```python
from build123d import *

# Parameters (mm, degrees)
ESQUISSE1_R                 = 20.5
ESQUISSE1_R_2               = 18.5
BOSS_EXTRU_1_DEPTH          = 20
BOSS_EXTRU_2_START          = 10
ESQUISSE2_R                 = 20.5
BOSS_EXTRU_2_DEPTH          = 10
BOSS_EXTRU_4_DEPTH          = 5
BOSS_EXTRU_5_DEPTH          = 10
TROU_TARAUD_M41_D           = 3.3
TROU_TARAUD_M41_CSINK_D     = 4.05
TROU_TARAUD_M41_CSINK_ANGLE = 90


with BuildPart() as part:
    # Esquisse1 → Boss.-Extru.1 (new body)
    with BuildSketch(Plane.XY):
        Circle(ESQUISSE1_R)
        Circle(ESQUISSE1_R_2, mode=Mode.SUBTRACT)
    extrude(amount=BOSS_EXTRU_1_DEPTH)

    # Esquisse2 → Boss.-Extru.2 (add)
    with BuildSketch(Plane(origin=(0, 0, 0), x_dir=(-1, 0, 0), z_dir=(0, 0, -1)).offset(BOSS_EXTRU_2_START)):
        Circle(ESQUISSE2_R)
    extrude(amount=-BOSS_EXTRU_2_DEPTH)



with BuildPart() as body_2:
    # Esquisse5 → Boss.-Extru.4 (new body)
    with BuildSketch(Plane(origin=(0, 20.5, 0), x_dir=(1, 0, 0), z_dir=(0, 1, 0))):
        Polygon((0, 0), (40, 0), (40, 10), (10, 10), (-40, 10), (-40, 0), align=None)
    extrude(amount=BOSS_EXTRU_4_DEPTH)


with BuildPart() as part_1:
    add(part.part)

    add(body_2.part)  # Boss.-Extru.5 merges body 2
    # Esquisse7 → Boss.-Extru.5 (add)
    with BuildSketch(Plane.XY.offset(-10)):
        with BuildLine():
            ThreePointArc((20.5, 0), (14.495689014, 14.495689014), (0, 20.5))
            Line((0, 20.5), (20.5, 20.5))
            Line((20.5, 20.5), (20.5, 0))
        make_face()
        with BuildLine():
            Line((-20.5, 20.5), (-20.5, 0))
            ThreePointArc((-20.5, 0), (-14.495689014, 14.495689014), (0, 20.5))
            Line((0, 20.5), (-20.5, 20.5))
        make_face()
    extrude(amount=BOSS_EXTRU_5_DEPTH)

    # Trou taraudé M41 (through all)
    with Locations(Plane(origin=(0, 20.5, 0), x_dir=(-1, 0, 0), z_dir=(0, -1, 0))):
        with Locations((-30.25, 5), (30.25, 5)):
            CounterSinkHole(TROU_TARAUD_M41_D / 2, TROU_TARAUD_M41_CSINK_D / 2, counter_sink_angle=TROU_TARAUD_M41_CSINK_ANGLE)


solid = part_1.part
```
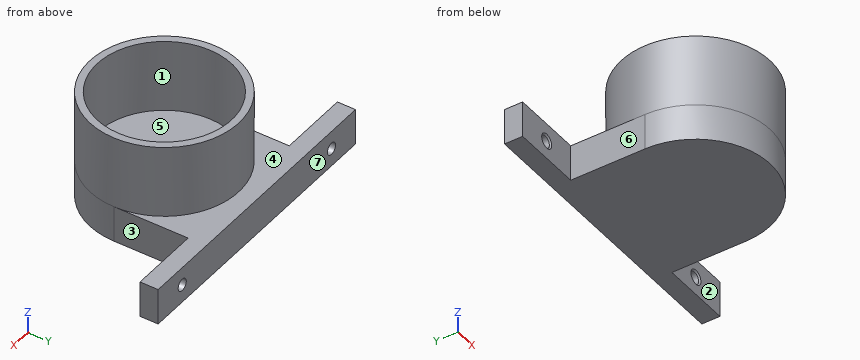
For this review, take the finished solid that the model builds, in its own axes (mm). Face numbers are marked on the shaded views. A direction names the side the tool comes from. Coordinates: 2 decimals unless noted, no trailing zeros. Order: outer loops, then holes, each group sorted by start corner. A loop starts at its lowest first (then second) coordinate and runs counter-clockwise, first axis right, second up. Notation, with made-up numbers: (-30.5, 9.25) -> (-6.5, 9.25) arc R14 cw to (-6.5, 19.25) -> close; hole circle Ø7 at (69.5, -36). An arc over 180 degrees is marked (long way). Answer as CSV lines item,"result".
Q1. We need section D-D (y = -10.5). State the section outline as (x, z) points, plus the area to 3 significant figures.
Model answer:
outline,"(-17.61, -10) -> (17.61, -10) -> (17.61, 20) -> (15.23, 20) -> (15.23, 0) -> (-15.23, 0) -> (-15.23, 20) -> (-17.61, 20) -> close"
area,"447 mm2"
Q2. For the marked faces 4, 5, 6 and 7, list the 3-axis set-ups (+Z, -Z, +X, -X, +Y, -Y) from which the entire face can be reached by the end or side of a thin tool; tool diameter is ignored.
Model answer:
face 4,"+Z, +Y"
face 5,"+Z"
face 6,"+Z, -Z, -X, -Y"
face 7,"+Z, -Z, +X, -X, +Y"
Q3. Clearance check with flat-ended pins moving along their axes: pin 1 Ø13 at (x, y) = (-9.5, 10.5) entering from +Z; pin 2 Ø3 at (y, z) = (10, -7) entering from +X; pin 3 Ø11 at (x, z) = (-29.5, -3.5) entering from -Y; pin 4 Ø8 at (y, z) = (14, -2.5) entering from -X. State where each tip first meets the part, or that it passes through.
Model answer:
pin 1,"stops at z = 20"
pin 2,"stops at x = 20.5"
pin 3,"stops at y = 20.5"
pin 4,"stops at x = -20.5"
Q4. Draft analysis for pull direction Y (two halves, no side actions). For the marked faces 1, 2 and 3, state which applies: released by +Y, released by -Y, zero draft, split by the parting line, or undercut.
Model answer:
face 1,"undercut"
face 2,"released by -Y"
face 3,"zero draft"
Q5. We need section A-A (z = -5). State the section outline as (x, y) points (3 decimals).
Model answer:
outline,"(-40, 20.5) -> (-32.275, 20.5) -> (-31.9, 20.875) -> (-31.9, 25.5) -> (-40, 25.5) -> close; (-28.6, 20.875) -> (-28.225, 20.5) -> (-20.5, 20.5) -> (-20.5, 0) arc R20.5 ccw to (20.5, 0) -> (20.5, 20.5) -> (28.225, 20.5) -> (28.6, 20.875) -> (28.6, 25.5) -> (-28.6, 25.5) -> close; (31.9, 20.875) -> (32.275, 20.5) -> (40, 20.5) -> (40, 25.5) -> (31.9, 25.5) -> close"
Q6. We need section C-C (x = 0). State the section outline as (y, z) points.
Model answer:
outline,"(-20.5, -10) -> (25.5, -10) -> (25.5, 0) -> (20.5, 0) -> (20.5, 20) -> (18.5, 20) -> (18.5, 0) -> (-18.5, 0) -> (-18.5, 20) -> (-20.5, 20) -> close"
Q7. We need section B-B (x = -30.25). State the section outline as (y, z) points (3 decimals), plus the area to 3 significant figures.
Model answer:
outline,"(20.5, -10) -> (25.5, -10) -> (25.5, -6.65) -> (20.875, -6.65) -> (20.5, -7.025) -> close; (20.5, -2.975) -> (20.875, -3.35) -> (25.5, -3.35) -> (25.5, 0) -> (20.5, 0) -> close"
area,"33.4 mm2"
Q8. Wall thickness on line 1 along X through (y, z) = (24.45, -5); line 2 along Y through (x, z) = (0, 5); line 3 along Z through (x, y) = (-30, 23): over which ranges is each line inside the solid? List them lowest first. Write a range as [from, to].
Model answer:
line 1,"x = [-40, -31.9], [-28.6, 28.6], [31.9, 40]"
line 2,"y = [-20.5, -18.5], [18.5, 20.5]"
line 3,"z = [-10, -6.63], [-3.37, 0]"
